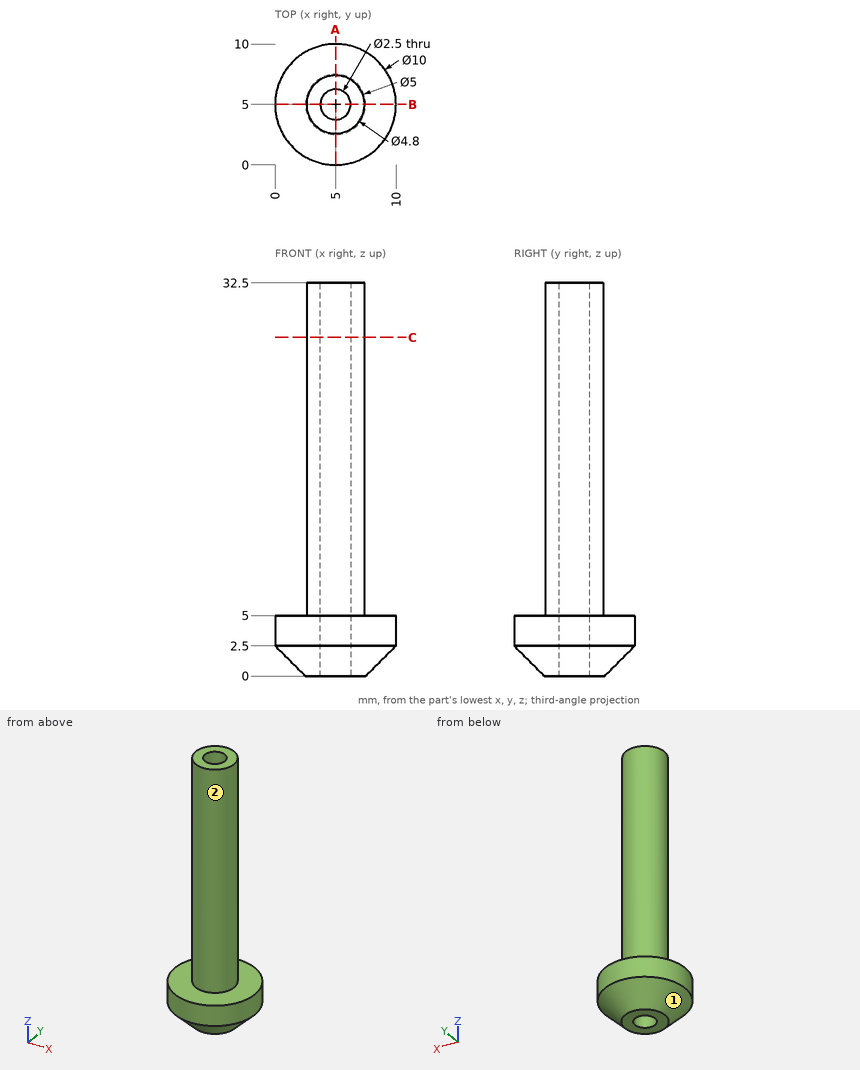
Geometry check sheet. Reference: drawing and pictorial views, mm from the part's lowest x, y, z. A direction names the side the tool comes from. Coordinates: 2 decimals unless noted, no trailing zeros. Write each loop counter-clockwise with the first axis right and the second up, starting at its lowest first coordinate (ties: lowest second). Pieces come first, ordered by that corner, then holes. Notation, with made-up numbers: M 71.25,4 L 106.25,4 A30 cw 106.25,26 Z; hole C -24.5,-8.5 d7. An arc over 180 degrees is marked long. Use one line per item in the form item = value.
Item 1: Set-up check for the marked faces 1 and 2: record each of +Z, -Z, +X, -X, +Y, -Y from which the full face is reachable in a straight line by a thin tool's end or side.
Answer below:
face_1 = -Z
face_2 = +Z
Item 2: Material ranges on L1, parallel to Y at x = 5, z = 22.5; L2, parallel to Y at x = 4.25, z = 13.5; L3, parallel to X at y = 6, z = 3.5, recorded low to high. Write a range as from..to.
Answer below:
L1 = 2.6..3.75, 6.25..7.4
L2 = 2.72..4, 6..7.28
L3 = 0.1..4.25, 5.75..9.9
Item 3: Sectioned sample at A-A, the plane x = 5. Record the cut outline in (y, z).
Answer below:
outline = M 0,2.5 L 2.5,0 L 3.75,0 L 3.75,32.5 L 2.6,32.5 L 2.6,5 L 0,5 Z; M 6.25,0 L 7.5,0 L 10,2.5 L 10,5 L 7.4,5 L 7.4,32.5 L 6.25,32.5 Z
Item 4: Sectioned sample at C-C, the plane z = 28. Record the cut outline in (x, y).
Answer below:
outline = C 5,5 d4.8; hole C 5,5 d2.5
Item 5: Gauge pin test, flat ends, axial feed: pin 1 Ø3 at (x, z) = (2, 14) entering from -Y; pin 2 Ø1 at (y, z) = (6.5, 19) entering from -X; pin 3 Ø3 at (x, z) = (5, 8) entering from +Y. Record the tip position at first contact, or that the pin passes through.
Answer below:
pin_1 = 3.13
pin_2 = 2.82
pin_3 = 7.4
